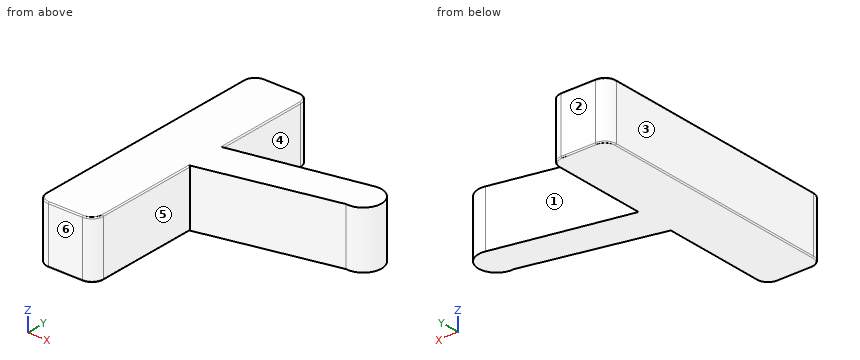
```python
from build123d import *

# Parameters (mm, degrees)
F1_DEPTH = 25
F4_R     = 0.5311269837
F5_R     = 0.5


# Not quite as in the source:
# - the program builds the solid bodies; features that only make, move or delete a surface that nothing else refers to are left out


with BuildPart() as f1:
    # F0 (on Top) → F1 (new body)
    with BuildSketch(Plane.XY):
        with BuildLine():
            Line((27.2940341383, 7.6065342873), (-29.9786943942, -4.0269889869))
            Line((-29.9786943942, -4.0269889869), (-29.9786943942, -21.0298318416))
            Line((-29.9786943942, -21.0298318416), (27.8906263411, -8.2031255588))
            ThreePointArc((27.8906263411, -8.2031255588), (36.9003542168, 0.052951297), (27.2940341383, 7.6065342873))
        make_face()
        with BuildLine():
            Line((-34.9786943942, 42.2088094056), (-50.0355128944, 42.2088094056))
            ThreePointArc((-50.0355128944, 42.2088094056), (-53.5710468003, 40.7443433115), (-55.0355128944, 37.2088094056))
            Line((-55.0355128944, 37.2088094056), (-55.0355128944, -66.7400610447))
            ThreePointArc((-55.0355128944, -66.7400610447), (-53.5710468003, -70.2755949506), (-50.0355128944, -71.7400610447))
            Line((-50.0355128944, -71.7400610447), (-34.9786943942, -71.7400610447))
            ThreePointArc((-34.9786943942, -71.7400610447), (-31.4431604883, -70.2755949506), (-29.9786943942, -66.7400610447))
            Line((-29.9786943942, -66.7400610447), (-29.9786943942, -21.0298318416))
            Line((-29.9786943942, -21.0298318416), (-29.9786943942, -4.0269889869))
            Line((-29.9786943942, -4.0269889869), (-29.9786943942, 37.2088094056))
            ThreePointArc((-29.9786943942, 37.2088094056), (-31.4431604883, 40.7443433115), (-34.9786943942, 42.2088094056))
        make_face()
    extrude(amount=F1_DEPTH)

    # F4
    f4_edges = [f1.edges().sort_by_distance(p)[0] for p in [
        (-29.978694, -43.884946, 25),
    ]]
    fillet(f4_edges, radius=F4_R)

    # F5
    f5_edges = [f1.edges().sort_by_distance(p)[0] for p in [
        (-29.978694, -43.884946, 0),
    ]]
    fillet(f5_edges, radius=F5_R)


solid = f1.part
```
Design review of the part built by this model. Coordinates are the model's own, in mm. Face numbers are marked on the shaded views. A direction names the side the tool comes from. Coordinates: 2 decimals unless noted, no trailing zeros. Write each loop counter-clockwise with the first axis right and the second up, starting at its lowest first coordinate (ties: lowest second). Pieces come first, ordered by that corner, then holes. Notation, with made-up numbers: M 27,87 L 35,87 A18 ccw 35,107 Z; hole C 81.5,-36.75 d4. An arc over 180 degrees is marked long. Answer as a JSON object with one key per item and string values.
Item 1: Add section D-D, the plane y = -15. Give the boundary of the cut face in (x, z), and give its area (3 significant figures).
Outcome:
{"outline": "M -55.04,0.5 A0.5 ccw -54.54,0 L -2.77,0 L -2.77,25 L -54.5,25 A0.53 ccw -55.04,24.47 Z", "area": "1,310 mm²"}
Item 2: Add section C-C, the plane x = -4. Give the boundary of the cut face in (y, z), and give its area (3 significant figures).
Outcome:
{"outline": "M -15.27,0 L 1.25,0 L 1.25,25 L -15.27,25 Z", "area": "413 mm²"}
Item 3: Machinability: for the marked faces 4, 5 and 6, which of the approach directions +Z, -Z, +X, -X, +Y, -Y give a long, thin tool a straight path to every point of the face, cutting with its end or side? Answer none if there is none.
Outcome:
{"face 4": "+Z, -Z, +Y", "face 5": "+Z, -Z, +X, -Y", "face 6": "+Z, -Z, +X, -X, -Y"}
Item 4: Draft analysis for pull direction X (two halves, no side actions). For the marked faces 1, 2 and 3, state which applies: pulls with the +X half, pulls with the -X half, needs draft (parallel to the pull), parting line crosses it, or undercut.
Outcome:
{"face 1": "undercut", "face 2": "needs draft", "face 3": "pulls with the -X half"}
Item 5: Add section A-A, the plane y = 11.5. Give the boundary of the cut face in (x, z), and give its area (3 significant figures).
Outcome:
{"outline": "M -55.04,0.5 A0.5 ccw -54.54,0 L -30.48,0 A0.5 ccw -29.98,0.5 L -29.98,24.47 A0.53 ccw -30.51,25 L -54.5,25 A0.53 ccw -55.04,24.47 Z", "area": "626 mm²"}
Item 6: Wall thickness on probe 1 along X at (y, z) = (-49, 1.5); probe 2 along Y at (x, z) = (28.5, 10.25); probe 3 along X at (y, z) = (-7, 14.75): over which ranges is each line inside the solid? List them lowest first.
Outcome:
{"probe 1": "-55.04 to -29.98", "probe 2": "-8.26 to 7.76", "probe 3": "-55.04 to 33.21"}
Item 7: Insertion check: pin 1 Ø12 at (x, z) = (9, 6.5) entering from +Y; pin 2 Ø2 at (x, z) = (3.5, 8.5) entering from -Y; pin 3 Ø12 at (y, z) = (11.5, 10.5) entering from +X. Each pin has a flat end and moves straight along its axis. Give the tip position at first contact, or say it passes through.
Outcome:
{"pin 1": "y = 5.11", "pin 2": "y = -13.83", "pin 3": "x = 34.48"}
Item 8: Add section B-B, the plane z = 12.5. Give the boundary of the cut face in (x, y), and give its area (3 significant figures).
Outcome:
{"outline": "M -55.04,-66.74 A5 ccw -50.04,-71.74 L -34.98,-71.74 A5 ccw -29.98,-66.74 L -29.98,-21.03 L 27.89,-8.2 A8.02 ccw long 27.29,7.61 L -29.98,-4.03 L -29.98,37.21 A5 ccw -34.98,42.21 L -50.04,42.21 A5 ccw -55.04,37.21 Z", "area": "3,900 mm²"}
